Source: CAD feature listing. Evaluate the final solid. Frame: model axes, mm. Face numbers are marked on the shaded views. Give positions to 0.01 mm unless a question says otherwise; leave off trailing zeros. Loops run counter-clockwise (first coordinate to the right, second up) from the corner with the lowest first, then second, coordinate; pieces in that order, holes last.
from build123d import *

# Parameters (mm, degrees)
F0_W      = 176
F0_H      = 146
F1_DEPTH  = 3
F2_W      = 50
F2_H      = 3
F2_W_2    = 3
F2_H_2    = 24
F2_W_3    = 109
F2_H_3    = 4
F2_R      = 1.25
F3_DEPTH  = 7
F3_FACE_W = 109
F3_FACE_H = 4
F4_R      = 1.25
F4_W      = 4
F4_H      = 98
F5_DEPTH  = 7
F6_W      = 2
F6_H      = 2
F7_DEPTH  = 176


# Not quite as in the source:
# - a feature names something its author has since deleted; it is built from what else it names


with BuildPart() as f1:
    # F0 (on Top) → F1 (new body)
    with BuildSketch(Plane.XY):
        with Locations((88, 73)):
            Rectangle(F0_W, F0_H)
    extrude(amount=F1_DEPTH)

    # F2 (on face) → F3 (join)
    with BuildSketch(Plane.XY.offset(3)):
        with Locations((53, 67.5)):
            Rectangle(F2_W, F2_H)
        with Locations((88.5, 38)):
            Rectangle(F2_W_2, F2_H_2)
        with Locations((60.5, 84)):
            Rectangle(F2_W_3, F2_H_3)
        with BuildLine():
            Line((0, 123), (6, 123))
            Line((6, 123), (21, 123))
            Line((21, 123), (21, 135))
            Line((21, 135), (44, 135))
            Line((44, 135), (44, 123))
            Line((44, 123), (71, 123))
            Line((71, 123), (71, 135))
            Line((71, 135), (94, 135))
            Line((94, 135), (94, 123))
            Line((94, 123), (121, 123))
            Line((121, 123), (121, 135))
            Line((121, 135), (144, 135))
            Line((144, 135), (144, 123))
            Line((144, 123), (170, 123))
            Line((170, 123), (170, 104))
            Line((170, 104), (162, 104))
            Line((162, 104), (162, 69))
            Line((162, 69), (160, 69))
            ThreePointArc((160, 69), (157, 66), (160, 63))
            Line((160, 63), (162, 63))
            Line((162, 63), (162, 21))
            Line((162, 21), (160, 21))
            ThreePointArc((160, 21), (157, 18), (160, 15))
            Line((160, 15), (162, 15))
            Line((162, 15), (162, 11))
            Line((162, 11), (0, 11))
            Line((0, 11), (0, 0))
            Line((0, 0), (176, 0))
            Line((176, 0), (176, 146))
            Line((176, 146), (0, 146))
            Line((0, 146), (0, 123))
        make_face()
        with Locations((13.75, 137)):
            Circle(F2_R, mode=Mode.SUBTRACT)
        with Locations((51.25, 137)):
            Circle(F2_R, mode=Mode.SUBTRACT)
        with Locations((63.75, 137)):
            Circle(F2_R, mode=Mode.SUBTRACT)
        with Locations((101.25, 137)):
            Circle(F2_R, mode=Mode.SUBTRACT)
        with Locations((113.75, 137)):
            Circle(F2_R, mode=Mode.SUBTRACT)
        with Locations((151.25, 137)):
            Circle(F2_R, mode=Mode.SUBTRACT)
    extrude(amount=F3_DEPTH)

    # F3_face (on face) + F4 (on face) → F5 (join)
    with BuildSketch(Plane(origin=(60.5, 84, 10), x_dir=(1, 0, 0), z_dir=(0, 0, 1))):
        Rectangle(F3_FACE_W, F3_FACE_H)
    with BuildSketch(Plane.XY.offset(10)):
        with BuildLine():
            Line((170, 146), (170, 123))
            Line((170, 123), (170, 104))
            Line((170, 104), (162, 104))
            Line((162, 104), (162, 69))
            Line((162, 69), (160, 69))
            ThreePointArc((160, 69), (157, 66), (160, 63))
            Line((160, 63), (162, 63))
            Line((162, 63), (162, 21))
            Line((162, 21), (160, 21))
            ThreePointArc((160, 21), (157, 18), (160, 15))
            Line((160, 15), (162, 15))
            Line((162, 15), (162, 11))
            Line((162, 11), (0, 11))
            Line((0, 11), (0, 0))
            Line((0, 0), (176, 0))
            Line((176, 0), (176, 146))
            Line((176, 146), (170, 146))
        make_face()
        with Locations((160, 18)):
            Circle(F4_R, mode=Mode.SUBTRACT)
        with Locations((170, 52)):
            Rectangle(F4_W, F4_H, mode=Mode.SUBTRACT)
        with Locations((160, 66)):
            Circle(F4_R, mode=Mode.SUBTRACT)
    extrude(amount=F5_DEPTH)

    # F6 (on face) → F7 (cut)
    with BuildSketch(Plane(origin=(0, 0, 0), x_dir=(0, -1, 0), z_dir=(-1, 0, 0))):
        with Locations((-145, 3)):
            Rectangle(F6_W, F6_H)
        with Locations((-1, 3)):
            Rectangle(F6_W, F6_H)
    extrude(amount=-F7_DEPTH, mode=Mode.SUBTRACT)


solid = f1.part
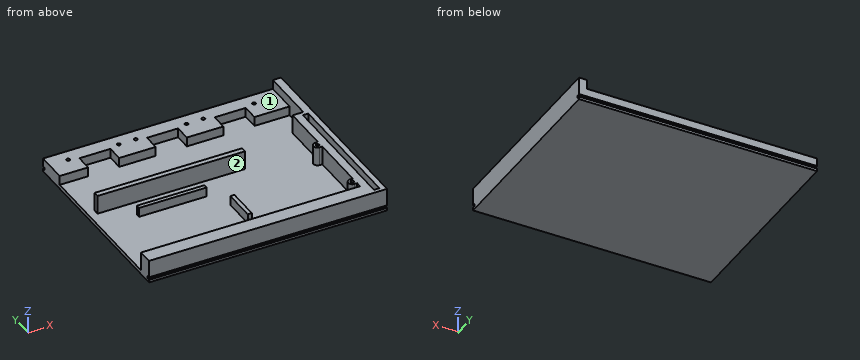
1) Contact query for flat-ended pins moving along their axis: P1, Ø0.6, axis at x = 86, y = 145, coming from the +Z side; P2, Ø5, axis at x = 136.5, y = 94.5, coming from the +Z side; P3, Ø3, axis at x = 35.5, z = 12, coming from the +Y side. Output: stop coordinate, or through.
Checks:
P1: stops at z = 10
P2: stops at z = 3
P3: stops at y = 86
2) Ray query, probe 1 along Y at (x, z) = (160, 13.75); probe 2 along Y at (x, z) = (101.25, 5); probe 3 along X at (y, z) = (66, 11.75). Return the intervals inside material, ascending.
Checks:
probe 1: y = 0 to 11, 15 to 16.75, 19.25 to 21, 63 to 64.75, 67.25 to 69
probe 2: y = 0 to 11, 82 to 86, 123 to 135.75, 138.25 to 146
probe 3: x = 157 to 158.75, 161.25 to 168, 172 to 176
3) Pull-direction query (Y, two-part tool) for the marked faces 1 and 2; classes: released by +Y, released by -Y, zero draft, split by the parting line, or undercut.
Checks:
face 1: zero draft
face 2: undercut
4) Cut plane A-A (z = 12.25). Return loops of the section in (x, y).
Checks:
outline: (0, 0) - (176, 0) - (176, 146) - (170, 146) - (170, 104) - (162, 104) - (162, 69) - (160, 69) arc R3 ccw to (160, 63) - (162, 63) - (162, 21) - (160, 21) arc R3 ccw to (160, 15) - (162, 15) - (162, 11) - (0, 11) - close; (6, 82) - (115, 82) - (115, 86) - (6, 86) - close; hole circle Ø2.5 at (160, 18); hole circle Ø2.5 at (160, 66); hole (168, 3) - (172, 3) - (172, 101) - (168, 101) - close
5) Cut plane D-D (y = 127). Return loops of the section in (x, z).
Checks:
outline: (0, 0) - (176, 0) - (176, 17) - (170, 17) - (170, 10) - (144, 10) - (144, 3) - (121, 3) - (121, 10) - (94, 10) - (94, 3) - (71, 3) - (71, 10) - (44, 10) - (44, 3) - (21, 3) - (21, 10) - (0, 10) - close
6) Cut plane C-C (x = 47.5). Return loops of the section in (y, z), and give its area (3 significant figures).
Checks:
outline: (0, 0) - (146, 0) - (146, 2) - (144, 2) - (144, 4) - (146, 4) - (146, 10) - (123, 10) - (123, 3) - (86, 3) - (86, 17) - (82, 17) - (82, 3) - (69, 3) - (69, 10) - (66, 10) - (66, 3) - (11, 3) - (11, 17) - (0, 17) - (0, 4) - (2, 4) - (2, 2) - (0, 2) - close
area: 822 mm2
7) Cut plane B-B (y = 46.5). Return loops of the section in (x, z), and give its area (3 significant figures).
Checks:
outline: (0, 0) - (176, 0) - (176, 17) - (172, 17) - (172, 10) - (168, 10) - (168, 17) - (162, 17) - (162, 3) - (90, 3) - (90, 10) - (87, 10) - (87, 3) - (0, 3) - close
area: 717 mm2
